```python
from build123d import *

# Parameters (mm, degrees)
SKETCH1_W           = 11.6
SKETCH1_H           = 16.6
BOSS_EXTRUDE1_DEPTH = 0.3
FILLET1_R           = 2
BOSS_EXTRUDE2_DEPTH = 1.2
BOSS_EXTRUDE3_DEPTH = 1
FILLET2_R           = 1


with BuildPart() as part:
    # Sketch1 → Boss-Extrude1 (new body)
    with BuildSketch(Plane.XY):
        Rectangle(SKETCH1_W, SKETCH1_H)
    extrude(amount=BOSS_EXTRUDE1_DEPTH)

    # Fillet1
    fillet1_edges = [part.edges().sort_by_distance(p)[0] for p in [
        (-5.8, 8.3, 0.15),
        (5.8, 8.3, 0.15),
    ]]
    fillet(fillet1_edges, radius=FILLET1_R)

    # Sketch2 → Boss-Extrude2 (add)
    with BuildSketch(Plane(origin=(0, 0, 0), x_dir=(-1, 0, 0), z_dir=(0, 0, -1))):
        with BuildLine():
            Line((-5.8, -8.3), (-5.8, 6.3))
            ThreePointArc((-5.8, 6.3), (-5.214213562, 7.714213562), (-3.8, 8.3))
            Line((-3.8, 8.3), (3.8, 8.3))
            ThreePointArc((3.8, 8.3), (5.214213562, 7.714213562), (5.8, 6.3))
            Line((5.8, 6.3), (5.8, -8.3))
            Line((5.8, -8.3), (-5.8, -8.3))
        make_face()
        with BuildLine():
            Line((-5, -7.5), (-5, 6.3))
            ThreePointArc((-5, 6.3), (-4.648528137, 7.148528137), (-3.8, 7.5))
            Line((-3.8, 7.5), (3.8, 7.5))
            ThreePointArc((3.8, 7.5), (4.648528137, 7.148528137), (5, 6.3))
            Line((5, 6.3), (5, -7.5))
            Line((5, -7.5), (-5, -7.5))
        make_face(mode=Mode.SUBTRACT)
    extrude(amount=BOSS_EXTRUDE2_DEPTH)

    # Sketch3 → Boss-Extrude3 (add)
    with BuildSketch(Plane(origin=(0, 0, -1.2), x_dir=(-1, 0, 0), z_dir=(0, 0, -1))):
        with BuildLine():
            Line((-8, 6.3), (-8, -10.5))
            Line((-8, -10.5), (2.8, -10.5))
            Line((2.8, -10.5), (2.8, -8.3))
            Line((2.8, -8.3), (5.8, -8.3))
            Line((5.8, -8.3), (5.8, -7.3))
            Line((5.8, -7.3), (8, -7.3))
            Line((8, -7.3), (8, 6.3))
            ThreePointArc((8, 6.3), (6.769848481, 9.269848481), (3.8, 10.5))
            Line((3.8, 10.5), (-3.8, 10.5))
            ThreePointArc((-3.8, 10.5), (-6.769848481, 9.269848481), (-8, 6.3))
        make_face()
        with BuildLine():
            Line((-5, 6.3), (-5, -7.5))
            Line((-5, -7.5), (5, -7.5))
            Line((5, -7.5), (5, 6.3))
            ThreePointArc((5, 6.3), (4.648528137, 7.148528137), (3.8, 7.5))
            Line((3.8, 7.5), (-3.8, 7.5))
            ThreePointArc((-3.8, 7.5), (-4.648528137, 7.148528137), (-5, 6.3))
        make_face(mode=Mode.SUBTRACT)
    extrude(amount=BOSS_EXTRUDE3_DEPTH)

    # Fillet2
    fillet2_edges = [part.edges().sort_by_distance(p)[0] for p in [
        (8, -10.5, -1.7),
        (-2.8, -10.5, -1.7),
        (-8, -7.3, -1.7),
    ]]
    fillet(fillet2_edges, radius=FILLET2_R)


solid = part.part
```
Read the model definition and answer for the solid it produces. Units are mm, in the model's axes. A direction names the side the tool comes from. Coordinates: 2 decimals unless noted, no trailing zeros. Order: outer loops, then holes, each group sorted by start corner. A loop starts at its lowest first (then second) coordinate and runs counter-clockwise, first axis right, second up. Notation, with made-up numbers: (84.5, -12.75) - (125.5, -12.75) arc R23 cw to (125.5, 15.25) - close; hole circle Ø5 at (54, 68). An arc over 180 degrees is marked (long way). Answer as a JSON object with one key per item and string values. Group by question number.
Item 1: Section C-C (x = 1.25) is taken. Give the vertices of the cut face in (y, z), plus the area to 3 significant figures.
Item 2: The mould has two halves that part along X. Classify faces 5 (the face through (5.8, -1, 0)), 6 (the face through (0, 0, 0)), 7 (the face through (0, 10.5, -2)): +X half, -X half, draft (parallel to the pull), parting line (faces both ways), or undercut.
Item 3: Section A-A (z = -1.75) is taken. Give the vertices of the cut face in (x, y).
Item 4: Consider probe 1 along Y at (x, z) = (-1.75, -1.15); probe 2 along X at (y, z) = (2, -0.35); probe 3 along Y at (x, z) = (1, -1.85). Determine where each line is inside the solid, lowest interval first. Write a range as from..to.
Item 5: Section B-B (y = 5.5) is taken. Give the vertices of the cut face in (x, z).
Item 6: Section D-D (z = -0.75) is taken. Give the vertices of the cut face in (x, y), plus the area to 3 significant figures.
Item 7: Flat-ended cylindrical pins translate along their axes: P1, Ø0.8, axis at x = -6.5, z = -1.5, coming from the -Y side; P2, Ø0.5, axis at y = -9, z = -1.5, coming from the -X side; P3, Ø0.7, axis at y = 0.5, z = -0.5, coming from the +X side. Find the tip coordinate at first contact, or state that the pin passes through.
Item 8: A tool of negligible diameter and unlimited length cuts with its end or side. For faces 1 (the face through (5.23, 7.7, -0.44)), 2 (the face through (-5, -1, -1)), 3 (the face through (-5.2, 7.73, -0.44)), 4 (the face through (0, 8.3, 0)), from which of +Z, -Z, +X, -X, +Y, -Y can it reach the whole face along a straight path? Write none if from no direction.
Results are:
{
 "1": {"outline": "(-10.5, -2.2) - (-7.5, -2.2) - (-7.5, 0) - (7.5, 0) - (7.5, -2.2) - (10.5, -2.2) - (10.5, -1.2) - (8.3, -1.2) - (8.3, 0.3) - (-8.3, 0.3) - (-8.3, -1.2) - (-10.5, -1.2) - close", "area": "12.9 mm^2"},
 "2": {"face 5": "+X half", "face 6": "undercut", "face 7": "draft"},
 "3": {"outline": "(-8, -6.3) arc R1 ccw to (-7, -7.3) - (-5.8, -7.3) - (-5.8, -8.3) - (-2.8, -8.3) - (-2.8, -9.5) arc R1 ccw to (-1.8, -10.5) - (7, -10.5) arc R1 ccw to (8, -9.5) - (8, 6.3) arc R4.2 ccw to (3.8, 10.5) - (-3.8, 10.5) arc R4.2 ccw to (-8, 6.3) - close; hole (-5, -7.5) - (5, -7.5) - (5, 6.3) arc R1.2 ccw to (3.8, 7.5) - (-3.8, 7.5) arc R1.2 ccw to (-5, 6.3) - close"},
 "4": {"probe 1": "y = -8.3..-7.5, 7.5..8.3", "probe 2": "x = -5.8..-5, 5..5.8", "probe 3": "y = -10.5..-7.5, 7.5..10.5"},
 "5": {"outline": "(-8, -2.2) - (-5, -2.2) - (-5, 0) - (5, 0) - (5, -2.2) - (8, -2.2) - (8, -1.2) - (5.8, -1.2) - (5.8, 0.3) - (-5.8, 0.3) - (-5.8, -1.2) - (-8, -1.2) - close"},
 "6": {"outline": "(-5.8, -8.3) - (5.8, -8.3) - (5.8, 6.3) arc R2 ccw to (3.8, 8.3) - (-3.8, 8.3) arc R2 ccw to (-5.8, 6.3) - close; hole (-5, -7.5) - (5, -7.5) - (5, 6.3) arc R1.2 ccw to (3.8, 7.5) - (-3.8, 7.5) arc R1.2 ccw to (-5, 6.3) - close", "area": "41.5 mm^2"},
 "7": {"P1": "stops at y = -7.3", "P2": "stops at x = -2.8", "P3": "stops at x = 5.8"},
 "8": {"face 1": "+Z, +X, +Y", "face 2": "-Z", "face 3": "+Z, -X, +Y", "face 4": "+Z, +X, -X, +Y"}
}
